```python
from build123d import *

# Parameters (mm, degrees)
F2_R     = 4.443183
F3_DEPTH = 25.4
F4_R     = 17.399446
F5_DEPTH = 25.4


with BuildPart() as f1:
    # F0 (on Front) → F1 (revolve)
    with BuildSketch(Plane.XZ):
        Polygon((-63.626997, 0), (0, 0), (0, 11.046355), (-63.626997, 11.046355), (-54.990999, 5.204355), align=None)
    revolve(axis=Axis((0, 0, 5.523177), (0, 0, -1)))

    # F2 (on face) → F3 (cut)
    with BuildSketch(Plane(origin=(0, 0, 0), x_dir=(1, 0, 0), z_dir=(0, 0, -1))):
        with Locations((37.211001, 41.018352)):
            Circle(F2_R)
    extrude(amount=-F3_DEPTH, mode=Mode.SUBTRACT)

    # F4 (on face) → F5 (cut)
    with BuildSketch(Plane(origin=(0, 0, 0), x_dir=(1, 0, 0), z_dir=(0, 0, -1))):
        Circle(F4_R)
    extrude(amount=-F5_DEPTH, mode=Mode.SUBTRACT)


solid = f1.part
```
Source: CAD feature listing. Evaluate the final solid. Frame: model axes, mm. A direction names the side the tool comes from. Give positions to 0.01 mm unless a question says otherwise; leave off trailing zeros. Loops run counter-clockwise (first coordinate to the right, second up) from the corner with the lowest first, then second, coordinate; pieces in that order, holes last. Notation, with made-up numbers: (-16, -7) -> (20, -7) arc R29 cw to (20, 23) -> close; hole circle Ø7 at (83, -18). An arc over 180 degrees is marked (long way). Use a Markdown table: item, result. Add a question column.
(1) Ray query, line 1 (X direction, y = -44, z = 10.25); line 2 (Y direction, x = -16, z = 2.5); line 3 (Z direction, x = 56, y = 27). Return the intervals inside material, ascending.
(2) Access query for faces 1 (the face through (12.04, -54.21, 4.88)), 2 (the face through (33.69, -38.31, 5.45)). Directions: +Z, -Z, +X, -X, +Y, -Y. A direction counts if a zero-diameter tool reaches every point of the face in a straight line with its end or side. Return the directions, or none.
(3) Section query A-A (x = 0). Output: boundary loops of the cut face in (y, z).
(4) First-contact query: pin 1 Ø6 at (x, y) = (11.5, -37) entering from -Z; pin 2 Ø1 at (x, z) = (34.5, 4.5) entering from +Y; pin 3 Ø7 at (x, y) = (37.21, -41.02) entering from +Z; pin 4 Ø3 at (x, z) = (12, 7) entering from +Y. Flat tips, straight axial feed; report the tip coordinate or a pass-through.
(5) Pull-direction query (Z, two-part tool) for faces 3 (the face through (16.073, 6.664, 5.446)), 4 (the face through (13, -13, 11.046)), 5 (the face through (12.012, -54.093, 5.488)); classes: +Z half, -Z half, draft (parallel to the pull), parting line (faces both ways), or undercut.
(6) Section query C-C (z = 9.5). Output: boundary loops of the cut face in (x, y).
Checked values:
| question | item | result |
|---|---|---|
| 1 | line 1 | -44.32 to 33.92, 40.51 to 44.32 |
| 1 | line 2 | -57.29 to -6.84, 6.84 to 57.29 |
| 1 | line 3 | 0 to 0.88, 10.06 to 11.05 |
| 2 | face 1 | none |
| 2 | face 2 | +Z, -Z |
| 3 | outline | (-63.63, 0) -> (-17.4, 0) -> (-17.4, 11.05) -> (-63.63, 11.05) -> (-54.99, 5.2) -> close; (17.4, 0) -> (63.63, 0) -> (54.99, 5.2) -> (63.63, 11.05) -> (17.4, 11.05) -> close |
| 4 | pin 1 | z = 0 |
| 4 | pin 2 | y = 45.43 |
| 4 | pin 3 | through |
| 4 | pin 4 | y = 58.67 |
| 5 | face 3 | draft |
| 5 | face 4 | +Z half |
| 5 | face 5 | undercut |
| 6 | outline | circle Ø122.68 at (0, 0); hole circle Ø34.8 at (0, 0); hole circle Ø8.89 at (37.21, -41.02) |
